Autodesk Inventor part; units mm, degrees
ref_plane "YZ Plane" through (0, 0, 0) normal (1, 0, 0) x (0, 1, 0)
ref_plane "XZ Plane" through (0, 0, 0) normal (0, 1, 0) x (-1, 0, 0)
ref_plane "XY Plane" through (0, 0, 0) normal (0, 0, 1) x (1, 0, 0)
sketch "Sketch1" plane through (0, 0, 0) normal (0, 0, 1) x (1, 0, 0)
  circle A0 centre (0, 0) radius 15
  circle A1 centre (0, 0) radius 4
  dimension "d0" = 30
  dimension "d1" = 8
extrude "Extrusion1" add sketch "Sketch1" along normal blind 10
sketch "Sketch3" plane through (0, 0, 10) normal (0, 0, 1) x (1, 0, 0)
  line L0 (0, 0) -> (25, 0) construction
  arc A0 (18.8792, 0.8) -> (14.8792, 1.9) centre (12.94, -12.9741) ccw
  circle A1 centre (0, 0) radius 15
  arc A2 (18.8792, -0.8) -> (18.8792, 0.8) centre (-1.1048, 0) ccw
  arc A3 (14.8792, -1.9) -> (18.8792, -0.8) centre (12.94, 12.9741) ccw
  arc A4 (14.8792, -1.9) -> (14.8792, 1.9) centre (0, 0) ccw
  arc A5 (17.467, 7.2088) -> (13.332, 6.8744) centre (16.5971, -7.7659) ccw
  arc A6 (18.0142, 5.7053) -> (17.467, 7.2088) centre (-1.0382, -0.3779) ccw
  arc A7 (14.6317, 3.3036) -> (18.0142, 5.7053) centre (7.7223, 16.6175) ccw
  arc A8 (14.6317, 3.3036) -> (13.332, 6.8744) centre (0, 0) ccw
  arc A9 (13.9481, 12.7481) -> (10.1768, 11.0196) centre (18.2523, -1.6211) ccw
  arc A10 (14.9765, 11.5225) -> (13.9481, 12.7481) centre (-0.8463, -0.7102) ccw
  arc A11 (12.6194, 8.1087) -> (14.9765, 11.5225) centre (1.573, 18.2565) ccw
  arc A12 (12.6194, 8.1087) -> (10.1768, 11.0196) centre (0, 0) ccw
  arc A13 (8.7468, 16.7498) -> (5.7941, 13.8357) centre (17.7059, 4.7193) ccw
  arc A14 (10.1324, 15.9498) -> (8.7468, 16.7498) centre (-0.5524, -0.9568) ccw
  arc A15 (9.085, 11.9357) -> (10.1324, 15.9498) centre (-4.7659, 17.6935) ccw
  arc A16 (9.085, 11.9357) -> (5.7941, 13.8357) centre (0, 0) ccw
  arc A17 (2.4905, 18.7313) -> (0.7126, 14.9831) centre (15.024, 10.4905) ccw
  arc A18 (4.0662, 18.4534) -> (2.4905, 18.7313) centre (-0.1918, -1.088) ccw
  arc A19 (4.4549, 14.3232) -> (4.0662, 18.4534) centre (-10.53, 14.9964) ccw
  arc A20 (4.4549, 14.3232) -> (0.7126, 14.9831) centre (0, 0) ccw
  arc A21 (-4.0662, 18.4534) -> (-4.4549, 14.3232) centre (10.53, 14.9964) ccw
  arc A22 (-2.4905, 18.7313) -> (-4.0662, 18.4534) centre (0.1918, -1.088) ccw
  arc A23 (-0.7126, 14.9831) -> (-2.4905, 18.7313) centre (-15.024, 10.4905) ccw
  arc A24 (-0.7126, 14.9831) -> (-4.4549, 14.3232) centre (0, 0) ccw
  arc A25 (-10.1324, 15.9498) -> (-9.085, 11.9357) centre (4.7659, 17.6935) ccw
  arc A26 (-8.7468, 16.7498) -> (-10.1324, 15.9498) centre (0.5524, -0.9568) ccw
  arc A27 (-5.7941, 13.8357) -> (-8.7468, 16.7498) centre (-17.7059, 4.7193) ccw
  arc A28 (-5.7941, 13.8357) -> (-9.085, 11.9357) centre (0, 0) ccw
  arc A29 (-14.9765, 11.5225) -> (-12.6194, 8.1087) centre (-1.573, 18.2565) ccw
  arc A30 (-13.9481, 12.7481) -> (-14.9765, 11.5225) centre (0.8463, -0.7102) ccw
  arc A31 (-10.1768, 11.0196) -> (-13.9481, 12.7481) centre (-18.2523, -1.6211) ccw
  arc A32 (-10.1768, 11.0196) -> (-12.6194, 8.1087) centre (0, 0) ccw
  arc A33 (-18.0142, 5.7053) -> (-14.6317, 3.3036) centre (-7.7223, 16.6175) ccw
  arc A34 (-17.467, 7.2088) -> (-18.0142, 5.7053) centre (1.0382, -0.3779) ccw
  arc A35 (-13.332, 6.8744) -> (-17.467, 7.2088) centre (-16.5971, -7.7659) ccw
  arc A36 (-13.332, 6.8744) -> (-14.6317, 3.3036) centre (0, 0) ccw
  arc A37 (-18.8792, -0.8) -> (-14.8792, -1.9) centre (-12.94, 12.9741) ccw
  arc A38 (-18.8792, 0.8) -> (-18.8792, -0.8) centre (1.1048, 0) ccw
  arc A39 (-14.8792, 1.9) -> (-18.8792, 0.8) centre (-12.94, -12.9741) ccw
  arc A40 (-14.8792, 1.9) -> (-14.8792, -1.9) centre (0, 0) ccw
  arc A41 (-17.467, -7.2088) -> (-13.332, -6.8744) centre (-16.5971, 7.7659) ccw
  arc A42 (-18.0142, -5.7053) -> (-17.467, -7.2088) centre (1.0382, 0.3779) ccw
  arc A43 (-14.6317, -3.3036) -> (-18.0142, -5.7053) centre (-7.7223, -16.6175) ccw
  arc A44 (-14.6317, -3.3036) -> (-13.332, -6.8744) centre (0, 0) ccw
  arc A45 (-13.9481, -12.7481) -> (-10.1768, -11.0196) centre (-18.2523, 1.6211) ccw
  arc A46 (-14.9765, -11.5225) -> (-13.9481, -12.7481) centre (0.8463, 0.7102) ccw
  arc A47 (-12.6194, -8.1087) -> (-14.9765, -11.5225) centre (-1.573, -18.2565) ccw
  arc A48 (-12.6194, -8.1087) -> (-10.1768, -11.0196) centre (0, 0) ccw
  arc A49 (-8.7468, -16.7498) -> (-5.7941, -13.8357) centre (-17.7059, -4.7193) ccw
  arc A50 (-10.1324, -15.9498) -> (-8.7468, -16.7498) centre (0.5524, 0.9568) ccw
  arc A51 (-9.085, -11.9357) -> (-10.1324, -15.9498) centre (4.7659, -17.6935) ccw
  arc A52 (-9.085, -11.9357) -> (-5.7941, -13.8357) centre (0, 0) ccw
  arc A53 (-2.4905, -18.7313) -> (-0.7126, -14.9831) centre (-15.024, -10.4905) ccw
  arc A54 (-4.0662, -18.4534) -> (-2.4905, -18.7313) centre (0.1918, 1.088) ccw
  arc A55 (-4.4549, -14.3232) -> (-4.0662, -18.4534) centre (10.53, -14.9964) ccw
  arc A56 (-4.4549, -14.3232) -> (-0.7126, -14.9831) centre (0, 0) ccw
  arc A57 (4.0662, -18.4534) -> (4.4549, -14.3232) centre (-10.53, -14.9964) ccw
  arc A58 (2.4905, -18.7313) -> (4.0662, -18.4534) centre (-0.1918, 1.088) ccw
  arc A59 (0.7126, -14.9831) -> (2.4905, -18.7313) centre (15.024, -10.4905) ccw
  arc A60 (0.7126, -14.9831) -> (4.4549, -14.3232) centre (0, 0) ccw
  arc A61 (10.1324, -15.9498) -> (9.085, -11.9357) centre (-4.7659, -17.6935) ccw
  arc A62 (8.7468, -16.7498) -> (10.1324, -15.9498) centre (-0.5524, 0.9568) ccw
  arc A63 (5.7941, -13.8357) -> (8.7468, -16.7498) centre (17.7059, -4.7193) ccw
  arc A64 (5.7941, -13.8357) -> (9.085, -11.9357) centre (0, 0) ccw
  arc A65 (14.9765, -11.5225) -> (12.6194, -8.1087) centre (1.573, -18.2565) ccw
  arc A66 (13.9481, -12.7481) -> (14.9765, -11.5225) centre (-0.8463, 0.7102) ccw
  arc A67 (10.1768, -11.0196) -> (13.9481, -12.7481) centre (18.2523, 1.6211) ccw
  arc A68 (10.1768, -11.0196) -> (12.6194, -8.1087) centre (0, 0) ccw
  arc A69 (18.0142, -5.7053) -> (14.6317, -3.3036) centre (7.7223, -16.6175) ccw
  arc A70 (17.467, -7.2088) -> (18.0142, -5.7053) centre (-1.0382, 0.3779) ccw
  arc A71 (13.332, -6.8744) -> (17.467, -7.2088) centre (16.5971, 7.7659) ccw
  arc A72 (13.332, -6.8744) -> (14.6317, -3.3036) centre (0, 0) ccw
  point P0 (18.8952, 0)
  point P1 (17.7557, 6.4625)
  point P2 (14.4746, 12.1456)
  point P3 (9.4476, 16.3637)
  point P4 (3.2811, 18.6081)
  point P5 (-3.2811, 18.6081)
  point P6 (-9.4476, 16.3637)
  point P7 (-14.4746, 12.1456)
  point P8 (-17.7557, 6.4625)
  point P9 (-18.8952, 0)
  point P10 (-17.7557, -6.4625)
  point P11 (-14.4746, -12.1456)
  point P12 (-9.4476, -16.3637)
  point P13 (-3.2811, -18.6081)
  point P14 (3.2811, -18.6081)
  point P15 (9.4476, -16.3637)
  point P16 (14.4746, -12.1456)
  point P17 (17.7557, -6.4625)
  dimension "d8" = 25
  dimension "d9" = 15
  dimension "d10" = 1.6
  dimension "d11" = 20
  dimension "d12" = 4
  dimension "d13" = 1.1
  dimension "d14" = 15
  dimension "d15" = 1.1
  dimension "d16" = 4
  dimension "d19" = 360
extrude "Extrusion3" add sketch "Sketch3" against normal blind 10 contours A2 A3 A1 A0 | A1 A5 A6 A7 | A69 A70 A71 A1 | A1 A9 A10 A11 | A65 A66 A67 A1 | A1 A13 A14 A15 | A61 A62 A63 A1 | A1 A17 A18 A19 | A57 A58 A59 A1 | A1 A21 A22 A23 | A53 A54 A55 A1 | A1 A25 A26 A27 | A49 A50 A51 A1 | A1 A29 A30 A31 | A45 A46 A47 A1 | A1 A33 A34 A35 | A41 A42 A43 A1 | A1 A37 A38 A39
sketch "Sketch2" plane through (0, 0, 10) normal (0, 0, 1) x (1, 0, 0)
  circle A0 centre (9.2572, 1.6323) radius 1.5
  circle A1 centre (0, 0) radius 15 construction
  circle A2 centre (0, 0) radius 4 construction
  circle A3 centre (0, 0) radius 4 construction
  circle A4 centre (0, 0) radius 15 construction
  arc A5 (14.8792, 1.9) -> (14.6317, 3.3036) centre (0, 0) ccw
  line L0 (0, 0) -> (3.9392, 0.6946) construction
  line L1 (0, 0) -> (14.7721, 2.6047) construction
  dimension "d4" = 3
  dimension "d24" = 9.4
extrude "Extrusion2" cut sketch "Sketch2" against normal through all
properties part number "GA002" material "ABS Plastic"
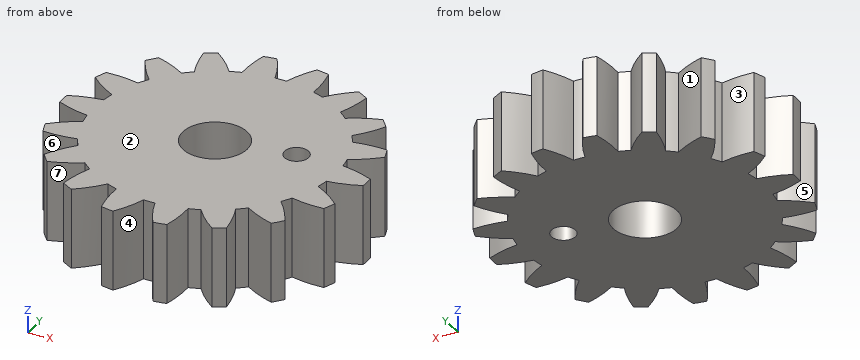
Can you work these out from the model? Positions are in its coordinate system, mm. Face numbers are marked on the shaded views. A direction names the side the tool comes from. Round coordinates to 2 decimals unless told otherwise and drop trailing zeros. Loops run counter-clockwise (first coordinate to the right, second up) from the corner with the lowest first, then second, coordinate; pieces in that order, holes last. Notation, with made-up numbers: M 40,2.5 L 51,2.5 A12 cw 51,14.5 Z; hole C 66.5,-13 d4. An arc over 180 degrees is marked long. Answer in a Markdown table with one row per item.
1. If we section it at B-B, the plane z = 4.5: Give the number of separate pieces and of enclosed holes in the cut face, plus the area to 3 significant figures.
Established:
| item | result |
|---|---|
| separate pieces | 1 |
| enclosed holes | 2 |
| area | 853 mm² |
2. I'm going to push flat-ended pins straight in: pin 1 Ø2 at (x, y) = (14.5, 2.5) entering from -Z; pin 2 Ø3 at (y, z) = (-5, 2) entering from +X; pin 3 Ø4 at (x, z) = (-7, 7) entering from +Y; pin 4 Ø1 at (y, z) = (-9, 2) entering from +X. Where does each tip first touch, or does it pass through?
Established:
| item | result |
|---|---|
| pin 1 | z = 0 |
| pin 2 | x = 18.01 |
| pin 3 | y = 16.75 |
| pin 4 | x = 13.75 |
3. Please list where these lines run through material, in increasing order: line 1 (Y direction, x = 0, z = 2.75); line 2 (X direction, y = -12, z = 2); line 3 (Y direction, x = 13.5, z = 3.25). Write a range as from..to.
Established:
| item | result |
|---|---|
| line 1 | -15..-4, 4..15 |
| line 2 | -14.6..-11.97, -9.11..9.11, 11.97..14.6 |
| line 3 | -12.61..-9.16, -6.91..6.91, 9.16..12.61 |
4. If we section it at A-A, the plane x = 0: Please give me the cut outline in (y, z), plus the area to 3 significant figures.
Established:
| item | result |
|---|---|
| outline | M -15,0 L -4,0 L -4,10 L -15,10 Z; M 4,0 L 15,0 L 15,10 L 4,10 Z |
| area | 220 mm² |
5. If we section it at C-C, the plane y = -5: Please give me the cut outline in (x, z).
Established:
| item | result |
|---|---|
| outline | M -17.21,0 L 17.21,0 L 17.21,10 L -17.21,10 Z |
6. On a 3-axis mill with a long thin cutter (end or side, diameter ignored), from which of +Z, -Z, +X, -X, +Y, -Y can I reach the whole of each face in a straight line? I mean the marked faces 5, 6 and 7. Say none if no direction works.
Established:
| item | result |
|---|---|
| face 5 | +Z, -Z, -X |
| face 6 | +Z, -Z |
| face 7 | +Z, -Z, -Y |
7. Thinking about a two-plate mould opening in Y: for the marked faces 1, 2, 3 and 4, which applies, pulls with the +Y half, pulls with the -Y half, needs draft (parallel to the pull), parting line crosses it, or undercut?
Established:
| item | result |
|---|---|
| face 1 | pulls with the +Y half |
| face 2 | needs draft |
| face 3 | undercut |
| face 4 | pulls with the -Y half |
